Check sheet for the modelled part. Datum: model origin and axes. Units: mm. A direction names the side the tool comes from. Coordinates: 2 decimals unless noted, no trailing zeros. Write each loop counter-clockwise with the first axis right and the second up, starting at its lowest first coordinate (ties: lowest second). Pieces come first, ordered by that corner, then holes. Notation, with made-up numbers: M -18.75,3.5 L 22.25,3.5 A24 ccw 22.25,29.5 Z; hole C 16.25,73 d6. An arc over 180 degrees is marked long. Answer as CSV lines item,"result".
from build123d import *

# Parameters (mm, degrees)
SKETCH1_R           = 9
BOSS_EXTRUDE1_DEPTH = 2
SKETCH2_R           = 5.75
BOSS_EXTRUDE2_DEPTH = 3
SKETCH3_R           = 6.75
BOSS_EXTRUDE3_DEPTH = 5
SKETCH4_R           = 5.75
BOSS_EXTRUDE4_DEPTH = 2
SKETCH5_R           = 8.5
BOSS_EXTRUDE5_DEPTH = 3


with BuildPart() as part:
    # Sketch1 → Boss-Extrude1 (new body)
    with BuildSketch(Plane(origin=(0, 0, 0), x_dir=(1, 0, 0), z_dir=(0, 1, 0))):
        Circle(SKETCH1_R)
    extrude(amount=BOSS_EXTRUDE1_DEPTH)

    # Sketch2 → Boss-Extrude2 (add)
    with BuildSketch(Plane(origin=(0, 2, 0), x_dir=(1, 0, 0), z_dir=(0, 1, 0))):
        Circle(SKETCH2_R)
    extrude(amount=BOSS_EXTRUDE2_DEPTH)

    # Sketch3 → Boss-Extrude3 (add)
    with BuildSketch(Plane(origin=(0, 5, 0), x_dir=(1, 0, 0), z_dir=(0, 1, 0))):
        Circle(SKETCH3_R)
    extrude(amount=BOSS_EXTRUDE3_DEPTH)

    # Sketch4 → Boss-Extrude4 (add)
    with BuildSketch(Plane(origin=(0, 10, 0), x_dir=(1, 0, 0), z_dir=(0, 1, 0))):
        Circle(SKETCH4_R)
    extrude(amount=BOSS_EXTRUDE4_DEPTH)

    # Sketch5 → Boss-Extrude5 (add)
    with BuildSketch(Plane(origin=(0, 12, 0), x_dir=(1, 0, 0), z_dir=(0, 1, 0))):
        Circle(SKETCH5_R)
    extrude(amount=BOSS_EXTRUDE5_DEPTH)


solid = part.part
1) Section check C-C, the plane x = -6.5. Record the boundary of the cut face in (y, z).
Answer key:
outline,"M 0,-6.22 L 2,-6.22 L 2,6.22 L 0,6.22 Z; M 5,-1.82 L 10,-1.82 L 10,1.82 L 5,1.82 Z; M 12,-5.48 L 15,-5.48 L 15,5.48 L 12,5.48 Z"
2) Depth check by flat-ended pin: P1, Ø6, axis at y = 7, z = -5.5, coming from the +X side; P2, Ø4, axis at x = 2, z = 0.5, coming from the -Y side; P3, Ø6, axis at x = 7, y = 9, coming from the -Z side. Enter the tip coordinate at first touch or a pass-through.
Answer key:
P1,"stops at x = 6.27"
P2,"stops at y = 0"
P3,"stops at z = -5.44"
3) Mould release check, pull along Y, two halves, no side actions. Record for faces 4 (the face through (-1.172, 0.986, -8.923)), 5 (the face through (-0.75, 10.99, -5.7)), 6 (the face through (-0.75, 3.48, -5.7)), 7 (the face through (0, 15, 0)): pulls with the +Y half, pulls with the -Y half, needs draft (parallel to the pull), parting line crosses it, or undercut.
Answer key:
face 4,"needs draft"
face 5,"undercut"
face 6,"undercut"
face 7,"pulls with the +Y half"
4) Section check D-D, the plane y = 11.5. Record the boundary of the cut face in (x, z).
Answer key:
outline,"C 0,0 d11.5"
5) Thickness scan on line 1 along Y through (x, z) = (-1.25, -6); line 2 along Y through (x, z) = (-7, 2.25); line 3 along Y through (x, z) = (-4.75, -7.5). Record the ranges inside material, lowest first.
Answer key:
line 1,"y = 0 to 2, 5 to 10, 12 to 15"
line 2,"y = 0 to 2, 12 to 15"
line 3,"y = 0 to 2"
6) Section check A-A, the plane x = 0. Record the boundary of the cut face in (y, z), plus the area to 3 significant figures.
Answer key:
outline,"M 0,-9 L 2,-9 L 2,-5.75 L 5,-5.75 L 5,-6.75 L 10,-6.75 L 10,-5.75 L 12,-5.75 L 12,-8.5 L 15,-8.5 L 15,8.5 L 12,8.5 L 12,5.75 L 10,5.75 L 10,6.75 L 5,6.75 L 5,5.75 L 2,5.75 L 2,9 L 0,9 Z"
area,"212 mm2"
7) Tool access check on faces 1 (the face through (0, 0, 0)), 2 (the face through (4.57, 13.479, -7.167)), 3 (the face through (0, 2, 6)). Record the directions out of +Z, -Z, +X, -X, +Y, -Y that give a thin tool (end or side, any length) a straight path to the whole face; none if there is none.
Answer key:
face 1,"+Z, -Z, +X, -X, -Y"
face 2,"+Y"
face 3,"none"
8) Section check B-B, the plane z = 0. Record the boundary of the cut face in (x, y), plus the area to 3 significant figures.
Answer key:
outline,"M -9,0 L 9,0 L 9,2 L 5.75,2 L 5.75,5 L 6.75,5 L 6.75,10 L 5.75,10 L 5.75,12 L 8.5,12 L 8.5,15 L -8.5,15 L -8.5,12 L -5.75,12 L -5.75,10 L -6.75,10 L -6.75,5 L -5.75,5 L -5.75,2 L -9,2 Z"
area,"212 mm2"
